Read the model definition and answer for the solid it produces. Units are mm, in the model's axes. A direction names the side the tool comes from. Give positions to 0.01 mm unless a question says otherwise; leave off trailing zeros. Order: outer loops, then holes, each group sorted by start corner. A loop starts at its lowest first (then second) coordinate and runs counter-clockwise, first axis right, second up.
```python
from build123d import *

# Parameters (mm, degrees)
F0_W      = 25.4
F0_H      = 25.4
F1_DEPTH  = 25.4
F3_D      = 4.7752
F3_DEPTH  = 3.81
F3_TIP    = 1.434614814
F6_D      = 4.7752
F6_DEPTH  = 3.81
F6_TIP    = 1.434614814
F9_D      = 4.7752
F9_DEPTH  = 3.81
F9_TIP    = 1.434614814
F12_D     = 4.7752
F12_DEPTH = 3.81
F12_TIP   = 1.434614814
F15_D     = 4.7752
F15_DEPTH = 3.81
F15_TIP   = 1.434614814
F18_D     = 4.7752
F18_DEPTH = 3.81
F18_TIP   = 1.434614814


with BuildPart() as f1:
    # F0 (on Top) → F1 (new body)
    with BuildSketch(Plane.XY):
        with Locations((12.7, 12.7)):
            Rectangle(F0_W, F0_H)
    extrude(amount=F1_DEPTH)

    # F3
    with Locations(Plane(origin=(0, 0, 0), x_dir=(1, 0, 0), z_dir=(0, 0, -1))):
        with Locations((12.5505877659, -13.2636902854)):
            Hole(F3_D / 2, depth=F3_DEPTH)
            with Locations((0, 0, -(F3_DEPTH + F3_TIP / 2))):  # 118° drill point
                Cone(0, F3_D / 2, F3_TIP, mode=Mode.SUBTRACT)

    # F6
    with Locations(Plane.XY.offset(25.4)):
        with Locations((7.7443891205, 20.0160127133), (17.0726701617, 20.0160127133), (17.0726701617, 13.5710183531), (7.7443891205, 13.5710183531), (17.0726701617, 6.6172094084), (7.7443891205, 6.6172094084)):
            Hole(F6_D / 2, depth=F6_DEPTH)
            with Locations((0, 0, -(F6_DEPTH + F6_TIP / 2))):  # 118° drill point
                Cone(0, F6_D / 2, F6_TIP, mode=Mode.SUBTRACT)

    # F9
    with Locations(Plane.YZ.offset(25.4)):
        with Locations((7.701497525, 17.8275406361), (18.2554014027, 17.8275406361), (18.2554014027, 6.9883959368), (7.701497525, 6.9883959368)):
            Hole(F9_D / 2, depth=F9_DEPTH)
            with Locations((0, 0, -(F9_DEPTH + F9_TIP / 2))):  # 118° drill point
                Cone(0, F9_D / 2, F9_TIP, mode=Mode.SUBTRACT)

    # F12
    with Locations(Plane(origin=(0, 0, 0), x_dir=(0, -1, 0), z_dir=(-1, 0, 0))):
        with Locations((-21.512749598, 21.4167089134), (-12.6499123884, 12.5934386103), (-4.6466261932, 4.6258819755)):
            Hole(F12_D / 2, depth=F12_DEPTH)
            with Locations((0, 0, -(F12_DEPTH + F12_TIP / 2))):  # 118° drill point
                Cone(0, F12_D / 2, F12_TIP, mode=Mode.SUBTRACT)

    # F15
    with Locations(Plane.XZ):
        with Locations((5.7652813432, 5.7883422565), (17.8275406361, 17.898850143)):
            Hole(F15_D / 2, depth=F15_DEPTH)
            with Locations((0, 0, -(F15_DEPTH + F15_TIP / 2))):  # 118° drill point
                Cone(0, F15_D / 2, F15_TIP, mode=Mode.SUBTRACT)

    # F18
    with Locations(Plane(origin=(0, 25.4, 0), x_dir=(-1, 0, 0), z_dir=(0, 1, 0))):
        with Locations((-20.2520862222, 18.9685039222), (-7.9867383465, 18.9685039222), (-14.5472735167, 13.2636902854), (-20.2520862222, 7.2736367583), (-7.9867383465, 7.2736367583)):
            Hole(F18_D / 2, depth=F18_DEPTH)
            with Locations((0, 0, -(F18_DEPTH + F18_TIP / 2))):  # 118° drill point
                Cone(0, F18_D / 2, F18_TIP, mode=Mode.SUBTRACT)


solid = f1.part
```
1) Given pin 1 (4.5 mm diameter, centred on y = 12.65, z = 12.59, fed in from -X); pin 2 (6 mm diameter, centred on y = 7.7, z = 17.83, fed in from -X); pin 3 (4 mm diameter, centred on x = 12.55, y = 13.26, fed in from -Z); pin 4 (3 mm diameter, centred on x = 14.55, z = 13.26, fed in from +Y), each flat-ended and moving along its own axis, determine where each tip first touches the part or whether it passes through.
Final values:
pin 1: stops at x = 3.89
pin 2: stops at x = 0
pin 3: stops at z = 4.04
pin 4: stops at y = 21.06
2) The part is cut by section A-A on x = 2.75. Determine the outline of the cut face in (y, z).
Final values:
outline: (0, 0) - (25.4, 0) - (25.4, 25.4) - (0, 25.4) - close; hole circle Ø4.78 at (4.65, 4.63); hole circle Ø4.78 at (12.65, 12.59); hole circle Ø4.78 at (21.51, 21.42)
3) For a pull along Z with two mould halves and no side action, classify faces 1 (the face through (23.47, 16.97, 9)), 2 (the face through (10.273, 12.547, 1.932)), 3 (the face through (20.405, 7.924, 7.338)), 4 (the face through (7.69, 13.982, 20.405)) as released by +Z, released by -Z, zero draft, split by the parting line, or undercut.
Final values:
face 1: undercut
face 2: zero draft
face 3: undercut
face 4: released by +Z
4) Consider L1, parallel to X at y = 12, z = 23.75; L2, parallel to X at y = 13, z = 24.5; L3, parallel to Y at x = 17.75, z = 23.75. Determine where each line is inside the solid, lowest interval first.
Final values:
L1: x = 0 to 5.95, 9.54 to 15.27, 18.87 to 25.4
L2: x = 0 to 5.43, 10.06 to 14.75, 19.39 to 25.4
L3: y = 0 to 4.33, 8.91 to 11.28, 15.86 to 17.73, 22.31 to 25.4
5) The part is cut by section B-B on x = 23.75. Determine the outline of the cut face in (y, z).
Final values:
outline: (0, 0) - (25.4, 0) - (25.4, 25.4) - (0, 25.4) - close; hole circle Ø4.78 at (7.7, 6.99); hole circle Ø4.78 at (7.7, 17.83); hole circle Ø4.78 at (18.26, 6.99); hole circle Ø4.78 at (18.26, 17.83)
6) A tool of negligible diameter and unlimited length cuts with its end or side. For faces 5 (the face through (23.468, 15.978, 18.545)), 6 (the face through (18.492, 23.468, 8.887)), 7 (the face through (9.64, 12.12, 23.47)), from which of +Z, -Z, +X, -X, +Y, -Y can it reach the whole face along a straight path? Write none if from no direction.
Final values:
face 5: +X
face 6: +Y
face 7: +Z
